Part model, mm, in its own coordinate system. A direction names the side the tool comes from. Give positions to 0.01 mm unless a question says otherwise; leave off trailing zeros. Order: outer loops, then holes, each group sorted by start corner. A loop starts at its lowest first (then second) coordinate and runs counter-clockwise, first axis right, second up. Notation, with made-up numbers: (1, -12) - (43, -12) arc R20 ccw to (43, -8) - close; hole circle Ø7 at (14, 39). An arc over 180 degrees is marked (long way). One line per item, written item: value.
Autodesk Inventor part; units mm, degrees
ref_plane "YZ Plane" through (0, 0, 0) normal (1, 0, 0) x (0, 1, 0)
ref_plane "XZ Plane" through (0, 0, 0) normal (0, 1, 0) x (-1, 0, 0)
ref_plane "XY Plane" through (0, 0, 0) normal (0, 0, 1) x (1, 0, 0)
sketch "Sketch1" plane through (0, 0, 0) normal (0, 0, 1) x (1, 0, 0)
  line L0 (0, 0) -> (36, 0)
  line L1 (36, 0) -> (36, 19)
  line L2 (36, 19) -> (0, 19)
  circle A0 centre (0, 19) radius 1.75
  circle A1 centre (0, 0) radius 1.75
  circle A2 centre (36, 0) radius 1.75
  circle A3 centre (36, 19) radius 1.75
  line L3 (0, 0) -> (0, -5)
  line L4 (0, -5) -> (40, -5)
  line L5 (0, -5) -> (-4, -5)
  line L6 (-4, -5) -> (-4, 25)
  line L7 (-4, 25) -> (40, 25)
  line L8 (40, 25) -> (40, -5)
  line L9 (36, 0) -> (36, 30)
  line L10 (36, 30) -> (0, 30)
  line L11 (18, 30) -> (48, 30)
  line L12 (48, 30) -> (48, 90)
  line L13 (48, 90) -> (-12, 90)
  line L14 (-12, 90) -> (-12, 30)
  line L15 (-4, 0) -> (-19, 0)
  line L16 (-19, 0) -> (-19, 95)
  line L17 (40, 0) -> (55, 0)
  line L18 (55, 0) -> (55, 95)
  line L19 (55, 95) -> (-19, 95)
  circle A4 centre (-12, 90) radius 1.75
  circle A5 centre (48, 90) radius 1.75
  circle A6 centre (-12, 30) radius 1.75
  circle A7 centre (48, 30) radius 1.75
  dimension "d0" = 36
  dimension "d1" = 19
  dimension "d2" = 3.5
  dimension "d3" = 3.5
  dimension "d4" = 3.5
  dimension "d5" = 3.5
  dimension "d6" = 5
  dimension "d7" = 40
  dimension "d8" = 4
  dimension "d9" = 30
  dimension "d10" = 30
  dimension "d11" = 30
  dimension "d12" = 60
  dimension "d13" = 60
  dimension "d14" = 15
  dimension "d15" = 95
  dimension "d16" = 15
  dimension "d17" = 3.5
  dimension "d18" = 3.5
  dimension "d19" = 3.5
  dimension "d20" = 3.5
extrude "Extrusion1" add sketch "Sketch1" along normal blind 5 contours A1 L3 L5 L6 L7 L9 A3 L1 A2 L0 | L0 A2 L1 A3 L9 L7 L8 L4 L3 A1 | L8 L7 L6 L15 L16 L19 L18 L17
sketch "Sketch2" plane through (0, 0, 5) normal (0, 0, 1) x (1, 0, 0)
  circle A0 centre (0, 19) radius 1.75
  circle A1 centre (0, 19) radius 3.5
  circle A2 centre (0, 0) radius 3.5
  circle A3 centre (36, 0) radius 1.75
  circle A4 centre (36, 0) radius 3.5
  circle A5 centre (36, 19) radius 3.5
  dimension "d23" = 7
  dimension "d24" = 7
  dimension "d25" = 7
  dimension "d26" = 7
extrude "Extrusion2" cut sketch "Sketch2" against normal blind 2.5
sketch "Sketch3" plane through (0, 0, 0) normal (0, 0, -1) x (-1, 0, 0)
  circle A0 centre (-48, 30) radius 1.75
  circle A1 centre (-48, 30) radius 3.5
  circle A2 centre (-48, 90) radius 1.75
  circle A3 centre (-48, 90) radius 3.5
  circle A4 centre (12, 90) radius 1.75
  circle A5 centre (12, 90) radius 3.5
  circle A6 centre (12, 30) radius 1.75
  circle A7 centre (12, 30) radius 3.5
  point P0 (0, 0)
  dimension "d29" = 7
  dimension "d30" = 7
  dimension "d31" = 7
  dimension "d32" = 7
extrude "Extrusion3" cut sketch "Sketch3" against normal blind 2.5
sketch "Sketch5" plane through (0, 0, 5) normal (0, 0, 1) x (1, 0, 0)
  circle A0 centre (0, 0) radius 1.75
  line L0 (0, 0) -> (0, 5)
  line L1 (0, 5) -> (5, 5)
  line L2 (5, 10) -> (5, 10)
  line L3 (10, 15) -> (25, 15)
  line L4 (30, 10) -> (30, 10)
  line L5 (25, 5) -> (10, 5)
  arc A1 (10, 15) -> (5, 10) centre (10, 10) ccw
  arc A2 (5, 10) -> (10, 5) centre (10, 10) ccw
  arc A3 (30, 10) -> (25, 15) centre (25, 10) ccw
  arc A4 (25, 5) -> (30, 10) centre (25, 10) ccw
  line L6 (-19, 0) -> (-14, 0)
  line L7 (-19, 0) -> (-4, 0)
  line L8 (-14, 0) -> (-14, 2)
  line L9 (-11, 2) -> (-10, 2)
  line L10 (-7, 5) -> (-7, 19)
  line L11 (-10, 22) -> (-11, 22)
  line L12 (-14, 19) -> (-14, 5)
  line L13 (-4, -5) -> (40, -5)
  line L14 (18, -5) -> (18, 1)
  arc A5 (-11, 22) -> (-14, 19) centre (-11, 19) ccw
  arc A6 (-7, 19) -> (-10, 22) centre (-10, 19) ccw
  arc A7 (-10, 2) -> (-7, 5) centre (-10, 5) ccw
  arc A8 (-14, 5) -> (-11, 2) centre (-11, 5) ccw
  line L15 (47, 2) -> (46, 2)
  line L16 (43, 5) -> (43, 19)
  line L17 (46, 22) -> (47, 22)
  line L18 (50, 19) -> (50, 5)
  arc A9 (50, 19) -> (47, 22) centre (47, 19) ccw
  arc A10 (46, 22) -> (43, 19) centre (46, 19) ccw
  arc A11 (43, 5) -> (46, 2) centre (46, 5) ccw
  arc A12 (47, 2) -> (50, 5) centre (47, 5) ccw
  line L19 (18, 0) -> (18, 95)
  line L20 (55, 95) -> (-19, 95)
  circle A13 centre (-12, 30) radius 1.75
  circle A14 centre (-12, 90) radius 1.75
  line L21 (-12, 30) -> (-12, 90)
  line L22 (-12, 60) -> (18, 60)
  line L23 (-12, 90) -> (18, 90)
  circle A15 centre (-12, 90) radius 3.5
  line L24 (-12, 90) -> (-7, 90)
  line L25 (-7, 90) -> (-7, 85)
  line L26 (-5, 85) -> (5.1716, 85)
  line L27 (-7, 83) -> (-7, 72.8284)
  line L28 (-3.5858, 71.4142) -> (6.5858, 81.5858)
  line L29 (18, 60) -> (18, 65)
  line L30 (18, 65) -> (13, 65)
  line L31 (11, 65) -> (0.8284, 65)
  line L32 (13, 67) -> (13, 77.1716)
  line L33 (9.5858, 78.5858) -> (-0.5858, 68.4142)
  arc A16 (6.5858, 81.5858) -> (5.1716, 85) centre (5.1716, 83) ccw
  arc A17 (-5, 85) -> (-7, 83) centre (-5, 83) ccw
  arc A18 (-7, 72.8284) -> (-3.5858, 71.4142) centre (-5, 72.8284) ccw
  arc A19 (-0.5858, 68.4142) -> (0.8284, 65) centre (0.8284, 67) ccw
  arc A20 (13, 77.1716) -> (9.5858, 78.5858) centre (11, 77.1716) ccw
  arc A21 (11, 65) -> (13, 67) centre (11, 67) ccw
  circle A22 centre (-12, 30) radius 3.5
  line L34 (-5, 35) -> (5.1716, 35)
  line L35 (-7, 37) -> (-7, 47.1716)
  line L36 (-3.5858, 48.5858) -> (6.5858, 38.4142)
  line L37 (11, 55) -> (0.8284, 55)
  line L38 (13, 53) -> (13, 42.8284)
  line L39 (9.5858, 41.4142) -> (-0.5858, 51.5858)
  arc A23 (5.1716, 35) -> (6.5858, 38.4142) centre (5.1716, 37) ccw
  arc A24 (-7, 37) -> (-5, 35) centre (-5, 37) ccw
  arc A25 (-3.5858, 48.5858) -> (-7, 47.1716) centre (-5, 47.1716) ccw
  arc A26 (0.8284, 55) -> (-0.5858, 51.5858) centre (0.8284, 53) ccw
  arc A27 (9.5858, 41.4142) -> (13, 42.8284) centre (11, 42.8284) ccw
  arc A28 (13, 53) -> (11, 55) centre (11, 53) ccw
  line L40 (41, 85) -> (30.8284, 85)
  line L41 (43, 83) -> (43, 72.8284)
  line L42 (39.5858, 71.4142) -> (29.4142, 81.5858)
  line L43 (25, 65) -> (35.1716, 65)
  line L44 (23, 67) -> (23, 77.1716)
  line L45 (26.4142, 78.5858) -> (36.5858, 68.4142)
  arc A29 (30.8284, 85) -> (29.4142, 81.5858) centre (30.8284, 83) ccw
  arc A30 (43, 83) -> (41, 85) centre (41, 83) ccw
  arc A31 (39.5858, 71.4142) -> (43, 72.8284) centre (41, 72.8284) ccw
  arc A32 (35.1716, 65) -> (36.5858, 68.4142) centre (35.1716, 67) ccw
  arc A33 (26.4142, 78.5858) -> (23, 77.1716) centre (25, 77.1716) ccw
  arc A34 (23, 67) -> (25, 65) centre (25, 67) ccw
  line L46 (43, 37) -> (43, 47.1716)
  arc A35 (41, 35) -> (43, 37) centre (41, 37) ccw
  arc A36 (43, 47.1716) -> (39.5858, 48.5858) centre (41, 47.1716) ccw
  line L47 (39.5858, 48.5858) -> (29.4142, 38.4142)
  line L48 (26.4142, 41.4142) -> (36.5858, 51.5858)
  line L49 (25, 55) -> (35.1716, 55)
  line L50 (23, 53) -> (23, 42.8284)
  line L51 (41, 35) -> (30.8284, 35)
  arc A37 (29.4142, 38.4142) -> (30.8284, 35) centre (30.8284, 37) ccw
  arc A38 (23, 42.8284) -> (26.4142, 41.4142) centre (25, 42.8284) ccw
  arc A39 (36.5858, 51.5858) -> (35.1716, 55) centre (35.1716, 53) ccw
  arc A40 (25, 55) -> (23, 53) centre (25, 53) ccw
  point P0 (5, 15)
  point P1 (30, 15)
  point P2 (30, 5)
  point P3 (-7, 2)
  point P4 (-7, 22)
  point P5 (-14, 22)
  point P6 (50, 2)
  point P7 (43, 2)
  point P8 (43, 22)
  point P9 (50, 22)
  point P10 (10, 85)
  point P11 (-7, 68)
  point P12 (-4, 65)
  point P13 (13, 82)
  point P14 (-7, 35)
  point P15 (10, 35)
  point P16 (-7, 52)
  point P17 (13, 55)
  point P18 (-4, 55)
  point P19 (13, 38)
  point P20 (43, 85)
  point P21 (26, 85)
  point P22 (43, 68)
  point P23 (23, 65)
  point P24 (40, 65)
  point P25 (23, 82)
  point P26 (26, 35)
  point P27 (23, 38)
  point P28 (43, 52)
  point P29 (40, 55)
  point P30 (43, 35)
  point P31 (23, 55)
  dimension "d40" = 5
  dimension "d41" = 5
  dimension "d42" = 10
  dimension "d43" = 25
  dimension "d44" = 5
  dimension "d45" = 5
  dimension "d46" = 2
  dimension "d47" = 7
  dimension "d48" = 20
  dimension "d49" = 3
  dimension "d50" = 5
  dimension "d51" = 5
  dimension "d52" = 17
  dimension "d53" = 17
  dimension "d54" = 5
  dimension "d55" = 5
  dimension "d56" = 17
  dimension "d57" = 17
  dimension "d58" = 2
extrude "Extrusion5" cut sketch "Sketch5" against normal through all contours L3 L19 L5 A2 A1 | L3 A3 A4 L5 L19 | A8 L12 A5 L11 A6 L10 A7 L9 | L15 A11 L16 A10 L17 A9 L18 A12 | L26 A16 L28 A18 L27 A17 | L31 A19 L33 A20 L32 A21 | A24 L35 A25 L36 A23 L34 | A28 L38 A27 L39 A26 L37 | A30 L41 A31 L42 A29 L40 | A34 L44 A33 L45 A32 L43 | A35 L51 A37 L47 A36 L46 | A38 L50 A40 L49 A39 L48
properties part number "nuccase_hold"
1) Slice it at D-D on x = -12. Write the cut outline in (y, z).
Answer:
outline: (0, 0) - (2.17, 0) - (2.17, 5) - (0, 5) - close; (21.83, 0) - (26.5, 0) - (26.5, 2.5) - (28.25, 2.5) - (28.25, 5) - (21.83, 5) - close; (31.75, 2.5) - (33.5, 2.5) - (33.5, 0) - (86.5, 0) - (86.5, 2.5) - (88.25, 2.5) - (88.25, 5) - (31.75, 5) - close; (91.75, 2.5) - (93.5, 2.5) - (93.5, 0) - (95, 0) - (95, 5) - (91.75, 5) - close
2) Slice it at C-C on y = 30. Write the cut outline in (x, z), then the cut area to 4 significant figures.
Answer:
outline: (-19, 0) - (-15.5, 0) - (-15.5, 2.5) - (-13.75, 2.5) - (-13.75, 5) - (-19, 5) - close; (-10.25, 2.5) - (-8.5, 2.5) - (-8.5, 0) - (44.5, 0) - (44.5, 2.5) - (46.25, 2.5) - (46.25, 5) - (-10.25, 5) - close; (49.75, 2.5) - (51.5, 2.5) - (51.5, 0) - (55, 0) - (55, 5) - (49.75, 5) - close
area: 317.5 mm2
3) Drop flat-ended pins along their axis: P1, Ø6.5, axis at x = 48, y = 90, coming from the -Z side; P2, Ø1.5, axis at y = -1.5, z = 1.5, coming from the +X side; P3, Ø6, axis at x = 28.5, y = 29, coming from the -Z side; P4, Ø2.5, axis at y = -2.5, z = 1.5, coming from the -X side. Give the stop position or say it passes through.
Answer:
P1: stops at z = 2.5
P2: stops at x = 40
P3: stops at z = 0
P4: stops at x = -4
4) Two-plate mould, pull along X, no slides. Class faces 1 (the face through (-19, 47, 2)), 2 (the face through (37.006, 66.204, 2.535)): pulls with the +X half, pulls with the -X half, needs draft (parallel to the pull), parting line crosses it, or undercut.
Answer:
face 1: pulls with the -X half
face 2: undercut
5) Slice it at A-A on y = 50.5. Write the cut outline in (x, z), then the cut area to 3 significant figures.
Answer:
outline: (-19, 0) - (0.5, 0) - (0.5, 5) - (-19, 5) - close; (13, 0) - (23, 0) - (23, 5) - (13, 5) - close; (35.5, 0) - (55, 0) - (55, 5) - (35.5, 5) - close
area: 245 mm2
6) Wall check: line 1 along X through (y, z) = (37, 3.15); line 2 along X through (y, z) = (90, 4.05); line 3 along Y through (x, z) = (-12, 1.2). Give the ranges that are in metal, low to high. Write a range as [from, to].
Answer:
line 1: x = [-19, -7], [7.17, 28.83], [43, 55]
line 2: x = [-19, -13.75], [-10.25, 46.25], [49.75, 55]
line 3: y = [0, 2.17], [21.83, 26.5], [33.5, 86.5], [93.5, 95]
7) Slice it at B-B on y = 10. Write the cut outline in (x, z).
Answer:
outline: (-19, 0) - (-14, 0) - (-14, 5) - (-19, 5) - close; (-7, 0) - (5, 0) - (5, 5) - (-7, 5) - close; (30, 0) - (43, 0) - (43, 5) - (30, 5) - close; (50, 0) - (55, 0) - (55, 5) - (50, 5) - close
8) Which spindle directions (+Z, -Z, +X, -X, +Y, -Y) get a long thin tool onto all of the face, cutting with end or side? Do faces 3 (the face through (35, 76, 3)), 4 (the face through (-4, -3, 2)), 5 (the face through (48.759, 86.583, 1.232)). Say none if no direction does.
Answer:
face 3: +Z, -Z
face 4: +Z, -Z, -X, -Y
face 5: -Z
